from build123d import *

# Parameters (mm, degrees)
SKETCH1_W           = 40.5
SKETCH1_H           = 45
BOSS_EXTRUDE1_DEPTH = 20
SKETCH2_R           = 2.5
BOSS_EXTRUDE2_DEPTH = 6
SKETCH3_R           = 2.548450287
CUT_EXTRUDE1_DEPTH  = 10


with BuildPart() as part:
    # Sketch1 → Boss-Extrude1 (new body)
    with BuildSketch(Plane.XY):
        Rectangle(SKETCH1_W, SKETCH1_H)
    extrude(amount=BOSS_EXTRUDE1_DEPTH)

    # Sketch2 → Boss-Extrude2 (add)
    with BuildSketch(Plane(origin=(0, 22.5, 0), x_dir=(1, 0, 0), z_dir=(0, 1, 0))):
        with Locations(Location((10.25, -10, 0), (0, 0, 90))):
            Circle(SKETCH2_R)
    extrude(amount=BOSS_EXTRUDE2_DEPTH)

    # Sketch3 → Cut-Extrude1 (cut)
    with BuildSketch(Plane(origin=(0, -22.5, 0), x_dir=(-1, 0, 0), z_dir=(0, -1, 0))):
        with Locations(Location((0, -10, 0), (0, 0, 90))):
            Circle(SKETCH3_R)
    extrude(amount=-CUT_EXTRUDE1_DEPTH, mode=Mode.SUBTRACT)


solid = part.part
Can you work these out from the model? Positions are in its coordinate system, mm. A direction names the side the tool comes from. Round coordinates to 2 decimals unless told otherwise and drop trailing zeros. Loops run counter-clockwise (first coordinate to the right, second up) from the corner with the lowest first, then second, coordinate; pieces in that order, holes last. Notation, with made-up numbers: (-7.5, 14) - (41.5, 14) arc R32 cw to (41.5, 50) - close; hole circle Ø9 at (34, 43). An arc over 180 degrees is marked (long way). Write item = value, one per line. Start each with the question number.
(1) If we section it at B-B (z = 10): Please give me the cut outline in (x, y).
(2) If we mould it in two halves opening along X, with no side actions, what happens to faces 1 (the face through (-1.551, -17.57, 12.022)), 2 (the face through (20.25, 0, 10)), 3 (the face through (0, -12.5, 10)), 4 (the face through (10, 28.5, 10))? For each: released by +X, released by -X, zero draft, split by the parting line, or undercut.
(3) If I drill on probe 1 along X at (y, z) = (-14.75, 10); probe 2 along Y at (x, z) = (11, 15.5); probe 3 along X at (y, z) = (-17, 11), over which ranges is the centre line in solid material (lowest first)? Write a range as [from, to].
(4) If we section it at C-C (x = 0): Please give me the cut outline in (y, z).
(5) If we section it at D-D (z = 17.5): Please give me the cut outline in (x, y).
(6) For faces 5 (the face through (12.7, 25.5, 10.5)), 6 (the face through (0, 0, 20)), which set-ups out of +Z, -Z, +X, -X, +Y, -Y let a thin tool reach every point of the face, with its end or its side?
(7) For P1, Ø6.5, axis at x = 0, z = 10, coming from the +Y side; P2, Ø2.5, axis at x = -0.5, z = 10.5, coming from the -Y side, each with a flat end and sliding along its axis, tell me the tip position at first contact or that it passes through.
(8) If we section it at A-A (x = 10.25): Please give me the cut outline in (y, z), and give its area (3 significant figures).
Ans:
q1.outline = (-20.25, -22.5) - (-2.55, -22.5) - (-2.55, -12.5) - (2.55, -12.5) - (2.55, -22.5) - (20.25, -22.5) - (20.25, 22.5) - (12.75, 22.5) - (12.75, 28.5) - (7.75, 28.5) - (7.75, 22.5) - (-20.25, 22.5) - close
q2.face_1 = undercut
q2.face_2 = released by +X
q2.face_3 = undercut
q2.face_4 = zero draft
q3.probe_1 = [-20.25, -2.55], [2.55, 20.25]
q3.probe_2 = [-22.5, 22.5]
q3.probe_3 = [-20.25, -2.34], [2.34, 20.25]
q4.outline = (-22.5, 0) - (22.5, 0) - (22.5, 20) - (-22.5, 20) - (-22.5, 12.55) - (-12.5, 12.55) - (-12.5, 7.45) - (-22.5, 7.45) - close
q5.outline = (-20.25, -22.5) - (20.25, -22.5) - (20.25, 22.5) - (-20.25, 22.5) - close
q6.face_5 = +Y
q6.face_6 = +Z, +X, -X, +Y, -Y
q7.P1 = 22.5
q7.P2 = -12.5
q8.outline = (-22.5, 0) - (22.5, 0) - (22.5, 7.5) - (28.5, 7.5) - (28.5, 12.5) - (22.5, 12.5) - (22.5, 20) - (-22.5, 20) - close
q8.area = 930 mm²
